Build history of the part. All positions in model axes, mm. A direction names the side the tool comes from. Give positions to 0.01 mm unless a question says otherwise; leave off trailing zeros. Write each loop counter-clockwise with the first axis right and the second up, starting at its lowest first coordinate (ties: lowest second). Pieces come first, ordered by that corner, then holes. Notation, with made-up numbers: (31, -25.5) -> (50, -25.5) arc R11 cw to (50, -10.5) -> close; hole circle Ø2 at (67.25, 68.5). An arc over 180 degrees is marked (long way). Put each result on its own line as item: value.
from build123d import *

# Parameters (mm, degrees)
SKETCH1_R                = 56
SKETCH1_R_2              = 28
BOSS_EXTRUDE1_DEPTH      = 31.5
BOSS_EXTRUDE2_REACH      = 246.59
BOSS_EXTRUDE2_END_RADIUS = 56
SKETCH2_W                = 63
SKETCH2_H                = 63
FILLET1_R                = 30
SKETCH3_R                = 28
BOSS_EXTRUDE3_DEPTH      = 50
SKETCH4_R                = 53.440477433
CUT_EXTRUDE1_DEPTH       = 80
FILLET2_R                = 20
BOSS_EXTRUDE4_DEPTH      = 50


with BuildPart() as part:
    # Sketch1 → Boss-Extrude1 (new, symmetric)
    with BuildSketch(Plane.XY):
        Circle(SKETCH1_R)
        Circle(SKETCH1_R_2, mode=Mode.SUBTRACT)
    extrude(amount=BOSS_EXTRUDE1_DEPTH, both=True)

    # Boss-Extrude2: up to this cylinder (the profile starts outside it)
    boss_extrude2_end = Plane(origin=(0, 0, 0), z_dir=(0, 0, -1)) * Cylinder(BOSS_EXTRUDE2_END_RADIUS, 606.18, mode=Mode.PRIVATE)
    # Sketch2 → Boss-Extrude2 (add, up to the surface)
    with BuildSketch(Plane(origin=(180, 0, 0), x_dir=(0, 0, -1), z_dir=(1, 0, 0)), mode=Mode.PRIVATE) as boss_extrude2_sk1:
        Rectangle(SKETCH2_W, SKETCH2_H)
    boss_extrude2_tool1 = extrude(boss_extrude2_sk1.sketch, amount=-BOSS_EXTRUDE2_REACH, mode=Mode.PRIVATE) - boss_extrude2_end
    add(boss_extrude2_tool1.solids().sort_by_distance((180, 0, 0))[0])

    # Fillet1
    fillet1_edges = [part.edges().sort_by_distance(p)[0] for p in [
        (46.300647944, -31.5, 0),
        (46.300647944, 31.5, 0),
    ]]
    fillet(fillet1_edges, radius=FILLET1_R)

    # Sketch3 → Boss-Extrude3 (add)
    with BuildSketch(Plane(origin=(180, 0, 0), x_dir=(0, 0, -1), z_dir=(1, 0, 0))):
        Circle(SKETCH3_R)
    extrude(amount=BOSS_EXTRUDE3_DEPTH)

    # Sketch4 → Cut-Extrude1 (cut)
    with BuildSketch(Plane(origin=(180, 0, 0), x_dir=(0, 0, -1), z_dir=(1, 0, 0))):
        Circle(SKETCH4_R)
        Polygon((18.186533479, -31.5), (36.373066959, 0), (18.186533479, 31.5), (-18.186533479, 31.5), (-36.373066959, 0), (-18.186533479, -31.5), align=None, mode=Mode.SUBTRACT)
    extrude(amount=-CUT_EXTRUDE1_DEPTH, mode=Mode.SUBTRACT)

    # Fillet2
    # the kernel refuses this fillet: 20 mm, written as the material it adds along each edge
    with BuildSketch(Plane(origin=(100, 74.801270189, -6.813466521), x_dir=(1, 0, 0), z_dir=(0, -0.8660254037844388, 0.4999999999999998))) as fillet2_piece_1_section:
        with BuildLine():
            CenterArc((FILLET2_R, FILLET2_R), FILLET2_R, 180, 90)
            Line((0, FILLET2_R), (0, 0))
            Line((0, 0), (FILLET2_R, 0))
        make_face()
    fillet2_piece_1 = extrude(amount=126.626933041, mode=Mode.PRIVATE)
    fillet2_piece_1 = split(fillet2_piece_1, bisect_by=Plane(origin=(105.889651232, 22.332439455, 31.5), z_dir=(0, 0, -1)), keep=Keep.TOP, mode=Mode.PRIVATE)
    fillet2_piece_1 = split(fillet2_piece_1, bisect_by=Plane(origin=(105.889651232, 31.5, 26.207106452), z_dir=(0, -1, 0)), keep=Keep.TOP, mode=Mode.PRIVATE)
    add(fillet2_piece_1)
    with BuildSketch(Plane(origin=(100, 34.860870628, 56.5), x_dir=(0, -0.4999999999999999, 0.8660254037844387), z_dir=(0, -0.8660254037844388, -0.4999999999999999))) as fillet2_piece_2_section:
        with BuildLine():
            CenterArc((FILLET2_R, -FILLET2_R), FILLET2_R, 90, 90)
            Line((0, -FILLET2_R), (0, 0))
            Line((0, 0), (FILLET2_R, 0))
        make_face()
    fillet2_piece_2 = extrude(amount=126.626933041, mode=Mode.PRIVATE)
    fillet2_piece_2 = split(fillet2_piece_2, bisect_by=Plane(origin=(105.889651233, -31.5, 26.207106452), z_dir=(0, 1, 0)), keep=Keep.TOP, mode=Mode.PRIVATE)
    fillet2_piece_2 = split(fillet2_piece_2, bisect_by=Plane(origin=(105.889651233, -22.332439456, 31.5), z_dir=(0, 0, -1)), keep=Keep.TOP, mode=Mode.PRIVATE)
    add(fillet2_piece_2)
    with BuildSketch(Plane(origin=(100, -74.801270189, 6.813466521), x_dir=(0, -0.4999999999999999, -0.8660254037844387), z_dir=(0, 0.8660254037844387, -0.49999999999999994))) as fillet2_piece_3_section:
        with BuildLine():
            CenterArc((FILLET2_R, -FILLET2_R), FILLET2_R, 90, 90)
            Line((0, -FILLET2_R), (0, 0))
            Line((0, 0), (FILLET2_R, 0))
        make_face()
    fillet2_piece_3 = extrude(amount=126.626933041, mode=Mode.PRIVATE)
    fillet2_piece_3 = split(fillet2_piece_3, bisect_by=Plane(origin=(105.889651233, -31.5, -26.207106452), z_dir=(0, 1, 0)), keep=Keep.TOP, mode=Mode.PRIVATE)
    fillet2_piece_3 = split(fillet2_piece_3, bisect_by=Plane(origin=(105.889651233, -22.332439456, -31.5), z_dir=(0, 0, 1)), keep=Keep.TOP, mode=Mode.PRIVATE)
    add(fillet2_piece_3)
    with BuildSketch(Plane(origin=(100, -34.860870628, -56.5), x_dir=(0, 0.49999999999999983, -0.8660254037844387), z_dir=(0, 0.8660254037844388, 0.4999999999999999))) as fillet2_piece_4_section:
        with BuildLine():
            CenterArc((FILLET2_R, -FILLET2_R), FILLET2_R, 90, 90)
            Line((0, -FILLET2_R), (0, 0))
            Line((0, 0), (FILLET2_R, 0))
        make_face()
    fillet2_piece_4 = extrude(amount=126.626933041, mode=Mode.PRIVATE)
    fillet2_piece_4 = split(fillet2_piece_4, bisect_by=Plane(origin=(105.889651233, 22.332439456, -31.5), z_dir=(0, 0, 1)), keep=Keep.TOP, mode=Mode.PRIVATE)
    fillet2_piece_4 = split(fillet2_piece_4, bisect_by=Plane(origin=(105.889651233, 31.5, -26.207106452), z_dir=(0, -1, 0)), keep=Keep.TOP, mode=Mode.PRIVATE)
    add(fillet2_piece_4)

    # Sketch5 → Boss-Extrude4 (add)
    with BuildSketch(Plane(origin=(180, 0, 0), x_dir=(0, 0, -1), z_dir=(1, 0, 0))):
        with BuildLine():
            Line((31.5, 8.440399562), (26.697558975, 8.440399562))
            ThreePointArc((26.697558975, 8.440399562), (28, 0), (26.697558975, -8.440399562))
            Line((26.697558975, -8.440399562), (31.5, -8.440399562))
            Line((31.5, -8.440399562), (31.5, 8.440399562))
        make_face()
    extrude(amount=BOSS_EXTRUDE4_DEPTH)


solid = part.part
1) Pin check, flat tips, straight feed: pin 1 (1 mm diameter, centred on y = -43.5, z = 12.5, fed in from -X); pin 2 (4 mm diameter, centred on y = 31, z = -1, fed in from -X); pin 3 (12 mm diameter, centred on x = 80, z = -15, fed in from +Y). Stop position of each tip, or through.
Filled sheet:
pin 1: x = -35.87
pin 2: x = -47.91
pin 3: y = 31.5
2) Slice it at A-A (x = 0). Write the cut outline in (y, z), plus the area to 3 significant figures.
Filled sheet:
outline: (-56, -31.5) -> (-28, -31.5) -> (-28, 31.5) -> (-56, 31.5) -> close; (28, -31.5) -> (56, -31.5) -> (56, 31.5) -> (28, 31.5) -> close
area: 3,530 mm2
3) Tool access for faces 1 (the flat face through (205, -8.44, -29)), 2 (the flat face through (205, 8.44, -29)), 3 (the flat face through (150.42, 20.13, 24.75)): list every direction of +Z, -Z, +X, -X, +Y, -Y with a clear straight run to the whole face (end or side of a thin tool).
Filled sheet:
face 1: -Z, +X, -Y
face 2: -Z, +X, +Y
face 3: +Z, +X, +Y
4) Slice it at B-B (z = 0). Write the cut outline in (x, y).
Filled sheet:
outline: (39.14, -40.05) arc R30 cw to (60.11, -31.5) -> (180, -31.5) -> (180, -28) -> (230, -28) -> (230, 28) -> (180, 28) -> (180, 31.5) -> (60.11, 31.5) arc R30 cw to (39.14, 40.05) arc R56 ccw (long way) to start; hole circle Ø56 at (0, 0)
5) Wall check: L1, parallel to Y at x = 0, z = 19; L2, parallel to Y at x = 82.5, z = 6.5; L3, parallel to X at y = -23, z = -23. Give the ranges that are in metal, low to high.
Filled sheet:
L1: -56 to -28, 28 to 56
L2: -31.5 to 31.5
L3: -51.06 to -15.97, 15.97 to 180
6) Slice it at C-C (y = 0). Write the cut outline in (x, z), plus the area to 3 significant figures.
Filled sheet:
outline: (-56, -31.5) -> (-28, -31.5) -> (-28, 31.5) -> (-56, 31.5) -> close; (28, -31.5) -> (230, -31.5) -> (230, 28) -> (180, 28) -> (180, 31.5) -> (28, 31.5) -> close
area: 14,300 mm2
7) Slice it at D-D (x = 144.5). Write the cut outline in (y, z).
Filled sheet:
outline: (-31.5, -18.19) -> (-8.44, -31.5) -> (8.44, -31.5) -> (31.5, -18.19) -> (31.5, 18.19) -> (8.44, 31.5) -> (-8.44, 31.5) -> (-31.5, 18.19) -> close
